For this review, take the finished solid that the model builds, in its own axes (mm). A direction names the side the tool comes from. Coordinates: 2 decimals unless noted, no trailing zeros. Loops run counter-clockwise (first coordinate to the right, second up) from the corner with the lowest first, then second, coordinate; pieces in that order, holes last. Notation, with made-up numbers: (3.5, -8) - (41.5, -8) arc R20 ccw to (41.5, 14) - close; hole circle Ø1 at (11, 69.25). An arc over 180 degrees is marked (long way). Answer as a JSON object with one key per item and string values. Group by question number.
Item 1: We need section C-C (y = 18). Give the boundary of the cut face in (x, z).
Item 2: To check wall thickness, follow line 1 (Y direction, x = -18, z = 0.5); line 2 (Y direction, x = -19.5, z = 0.5); line 3 (X direction, y = -1.5, z = 1.5). State the ranges of each line that lie inside material, in increasing order.
Item 3: Mouldability with a two-part tool opening along X and no side actions: class faces 3 (the flat face through (1, 19, 4)), 4 (the flat face through (0, 0, 0)) as released by +X, released by -X, zero draft, split by the parting line, or undercut.
Item 4: Tool access review of faces 1 (the flat face through (17.56, 0.01, 5.94)), 2 (the cylindrical face through (16.643, 17.013, 4.93)): name each direction out of +Z, -Z, +X, -X, +Y, -Y from which nothing blocks a thin tool from reaching the whole face with its end or side.
Item 5: We need section B-B (x = -8.5). Give the boundary of the cut face in (y, z).
Item 6: We need section A-A (y = 6). Give the boundary of the cut face in (x, z), then the cut area to 3 significant figures.
Item 7: Clearance check with flat-ended pins moving along their axes: pin 1 (1.5 mm diameter, centred on x = -12, z = 3.5, fed in from -Y); pin 2 (5 mm diameter, centred on x = 14, y = 13, fed in from +Z); pin 3 (5 mm diameter, centred on x = -15.5, z = 4.5, fed in from -Y); pin 4 (3 mm diameter, centred on x = -13.5, z = 6, fed in from +Y). State where each tip first meets the part, or that it passes through.
Autodesk Inventor part; units mm, degrees
ref_plane "YZ Plane" through (0, 0, 0) normal (1, 0, 0) x (0, 1, 0)
ref_plane "XZ Plane" through (0, 0, 0) normal (0, 1, 0) x (-1, 0, 0)
ref_plane "XY Plane" through (0, 0, 0) normal (0, 0, 1) x (1, 0, 0)
sketch "スケッチ1" plane through (0, 0, 0) normal (0, 0, 1) x (1, 0, 0)
  circle A0 centre (0, 0) radius 12
  dimension "d0" = 24
extrude "ハブ" add sketch "スケッチ1" along normal blind 2
sketch "スケッチ2" plane through (0, 0, 0) normal (0, 0, 1) x (1, 0, 0)
  circle A0 centre (0, 0) radius 25
  circle A1 centre (0, 0) radius 23.8
  dimension "d3" = 50
  dimension "d4" = 1.2
extrude "リム" add sketch "スケッチ2" along normal blind 10
sketch "スケッチ5" plane through (0, 0, 0) normal (1, 0, 0) x (0, 1, 0)
  line L0 (23.8, 10) -> (23.8, 0)
  line L1 (23.8, 10) -> (23.8, 0)
  line L2 (23.8, 0) -> (11.5, 0)
  line L3 (25, 0) -> (-25, 0)
  line L4 (11.5, 0) -> (11.5, 2)
  line L5 (11.5, 2) -> (23.8, 10)
  line L6 (12, 2) -> (-12, 2)
  point P0 (0, 0)
  point P1 (0, 0)
  dimension "d10" = 11.5
extrude "スポーク" add sketch "スケッチ5" along normal mid plane 2
pattern_circular "円形状パターン1" count 4 over 360 about axis through (0, 0, -10) along (0, 0, 1) of "スポーク"
sketch "スケッチ6" plane through (0, 0, 2) normal (0, 0, 1) x (1, 0, 0)
  circle A0 centre (0, 0) radius 8 construction
  line L0 (-13.4189, -13.4189) -> (13.4189, 13.4189) construction
  line L1 (-15.0493, 15.0493) -> (15.0493, -15.0493) construction
  line L2 (-16.6434, 0) -> (16.6434, 0) construction
  point P0 (5.6569, 5.6569)
  point P1 (-5.6569, 5.6569)
  point P2 (-5.6569, -5.6569)
  point P3 (5.6569, -5.6569)
  dimension "d16" = 16
  dimension "d17" = 45
  dimension "d18" = 45
hole "穴1" at (5.6569, 5.6569, 2) at (-5.6569, 5.6569, 2) at (-5.6569, -5.6569, 2) at (5.6569, -5.6569, 2) direction (0, 0, -1) diameter 3.2 end through all
equation "\"d18\" = d17"
properties part number "Wheel-D50A"
Check sheet entries:
{
 "1": {"outline": "(-17.35, 0) - (-15.57, 0) - (-15.57, 10) - (-17.35, 10) - close; (-1, 0) - (1, 0) - (1, 6.23) - (-1, 6.23) - close; (15.57, 0) - (17.35, 0) - (17.35, 10) - (15.57, 10) - close"},
 "2": {"line 1": "y = -17.35 to -15.57, -1 to 1, 15.57 to 17.35", "line 2": "y = -15.64 to -13.65, -1 to 1, 13.65 to 15.64", "line 3": "x = -24.95 to -23.75, -11.91 to 11.91, 23.75 to 24.95"},
 "3": {"face 3": "undercut", "face 4": "zero draft"},
 "4": {"face 1": "+Z", "face 2": "+Z, -Z"},
 "5": {"outline": "(-23.51, 0) - (-22.23, 0) - (-22.23, 10) - (-23.51, 10) - close; (-8.47, 0) - (8.47, 0) - (8.47, 2) - (-8.47, 2) - close; (22.23, 0) - (23.51, 0) - (23.51, 10) - (22.23, 10) - close"},
 "6": {"outline": "(-24.27, 0) - (-23.03, 0) - (-23.03, 10) - (-24.27, 10) - close; (-10.39, 0) - (-7.22, 0) - (-7.22, 2) - (-10.39, 2) - close; (-4.09, 0) - (4.09, 0) - (4.09, 2) - (-4.09, 2) - close; (7.22, 0) - (10.39, 0) - (10.39, 2) - (7.22, 2) - close; (23.03, 0) - (24.27, 0) - (24.27, 10) - (23.03, 10) - close", "area": "53.8 mm2"},
 "7": {"pin 1": "stops at y = -22.33", "pin 2": "passes through", "pin 3": "stops at y = -21.35", "pin 4": "stops at y = 21.93"}
}
